from build123d import *

# Parameters (mm, degrees)
BOSS_EXTRUDE1_DEPTH                             = 3
BOSS_EXTRUDE2_START                             = 10
SKETCH2_R                                       = 2
BOSS_EXTRUDE2_DEPTH                             = 10
FILLET2_R                                       = 2
CSK_FOR_M3_FLAT_HEAD_MACHINE_SCREW1_D           = 3.2
CSK_FOR_M3_FLAT_HEAD_MACHINE_SCREW1_CSINK_D     = 6.3
CSK_FOR_M3_FLAT_HEAD_MACHINE_SCREW1_CSINK_ANGLE = 90
BOSS_EXTRUDE3_DEPTH                             = 2
BOSS_EXTRUDE3_DEPTH_BACK                        = 4
SKETCH5_W                                       = 113
SKETCH5_H                                       = 2
SKETCH5_W_2                                     = 2
SKETCH5_H_2                                     = 58
CHAMFER1_SIZE                                   = 2
CHAMFER2_SIZE                                   = 0.5
SKETCH6_R                                       = 1.75
CUT_EXTRUDE1_DEPTH                              = 86.283351383
SKETCH7_R                                       = 4
SKETCH7_R_2                                     = 2.75
BOSS_EXTRUDE4_DEPTH                             = 1.5
CUT_EXTRUDE2_START                              = -4
SKETCH8_R                                       = 2.75
CUT_EXTRUDE2_DEPTH                              = 4


with BuildPart() as part:
    # Sketch1 → Boss-Extrude1 (new body)
    with BuildSketch(Plane.XY):
        with BuildLine():
            Line((-66.5, 44), (66.5, 44))
            ThreePointArc((66.5, 44), (70.035533906, 42.535533906), (71.5, 39))
            Line((71.5, 39), (71.5, -39))
            ThreePointArc((71.5, -39), (70.035533906, -42.535533906), (66.5, -44))
            Line((66.5, -44), (-66.5, -44))
            ThreePointArc((-66.5, -44), (-70.035533906, -42.535533906), (-71.5, -39))
            Line((-71.5, -39), (-71.5, 39))
            ThreePointArc((-71.5, 39), (-70.035533906, 42.535533906), (-66.5, 44))
        make_face()
    extrude(amount=BOSS_EXTRUDE1_DEPTH)

    # Sketch2 → Boss-Extrude2 (add)
    with BuildSketch(Plane(origin=(0, 0, 0), x_dir=(-1, 0, 0), z_dir=(0, 0, -1)).offset(BOSS_EXTRUDE2_START)):
        with BuildLine():
            Line((-66.5, 44), (66.5, 44))
            ThreePointArc((66.5, 44), (70.035533906, 42.535533906), (71.5, 39))
            Line((71.5, 39), (71.5, -39))
            ThreePointArc((71.5, -39), (70.035533906, -42.535533906), (66.5, -44))
            Line((66.5, -44), (-66.5, -44))
            ThreePointArc((-66.5, -44), (-70.035533906, -42.535533906), (-71.5, -39))
            Line((-71.5, -39), (-71.5, 39))
            ThreePointArc((-71.5, 39), (-70.035533906, 42.535533906), (-66.5, 44))
        make_face()
        with Locations((-66.5, 39)):
            Circle(SKETCH2_R, mode=Mode.SUBTRACT)
        with Locations(Location((66.5, 39, 0), (0, 0, 180))):
            Circle(SKETCH2_R, mode=Mode.SUBTRACT)
        with Locations((66.5, -39)):
            Circle(SKETCH2_R, mode=Mode.SUBTRACT)
        with Locations(Location((-66.5, -39, 0), (0, 0, 180))):
            Circle(SKETCH2_R, mode=Mode.SUBTRACT)
        with BuildLine():
            Line((-61.917424305, 41), (61.917424305, 41))
            Line((61.917424305, 41), (61.917424305, 37))
            ThreePointArc((61.917424305, 37), (64.673843213, 34.345416088), (68.5, 34.417424305))
            Line((68.5, 34.417424305), (68.5, -34.417424305))
            ThreePointArc((68.5, -34.417424305), (64.673843213, -34.345416088), (61.917424305, -37))
            Line((61.917424305, -37), (61.917424305, -41))
            Line((61.917424305, -41), (-61.917424305, -41))
            ThreePointArc((-61.917424305, -41), (-62.964466094, -35.464466094), (-68.5, -34.417424305))
            Line((-68.5, -34.417424305), (-68.5, 34.417424305))
            ThreePointArc((-68.5, 34.417424305), (-62.964466094, 35.464466094), (-61.917424305, 41))
        make_face(mode=Mode.SUBTRACT)
    extrude(amount=-BOSS_EXTRUDE2_DEPTH)

    # Fillet2
    fillet2_edges = [part.edges().sort_by_distance(p)[0] for p in [
        (-70.035533906, -42.535533906, 3),
        (0, -44, 3),
        (70.035533906, -42.535533906, 3),
        (71.5, 0, 3),
        (70.035533906, 42.535533906, 3),
        (0, 44, 3),
        (0, 41, 0),
        (68.5, 0, 0),
        (0, -41, 0),
        (-68.5, 0, 0),
        (-70.035533906, 42.535533906, 3),
        (-71.5, 0, 3),
    ]]
    fillet(fillet2_edges, radius=FILLET2_R)

    # CSK for M3 Flat Head Machine Screw1 (through all)
    with Locations(Plane.XY.offset(3)):
        with Locations((-66.5, 39), (66.5, 39), (66.5, -39), (-66.5, -39)):
            CounterSinkHole(CSK_FOR_M3_FLAT_HEAD_MACHINE_SCREW1_D / 2, CSK_FOR_M3_FLAT_HEAD_MACHINE_SCREW1_CSINK_D / 2, counter_sink_angle=CSK_FOR_M3_FLAT_HEAD_MACHINE_SCREW1_CSINK_ANGLE)

    # Sketch5 → Boss-Extrude3 (add, two sides: drawn at the far end of the back side and taken through both)
    with BuildSketch(Plane(origin=(0, 0, -10), x_dir=(-1, 0, 0), z_dir=(0, 0, -1)).offset(-BOSS_EXTRUDE3_DEPTH_BACK)):
        with Locations((0, 40)):
            Rectangle(SKETCH5_W, SKETCH5_H)
        with Locations((-67.5, 0)):
            Rectangle(SKETCH5_W_2, SKETCH5_H_2)
        with Locations((0, -40)):
            Rectangle(SKETCH5_W, SKETCH5_H)
        with Locations((67.5, 0)):
            Rectangle(SKETCH5_W_2, SKETCH5_H_2)
    extrude(amount=BOSS_EXTRUDE3_DEPTH + BOSS_EXTRUDE3_DEPTH_BACK)

    # Chamfer1
    chamfer1_edges = [part.edges().sort_by_distance(p)[0] for p in [
        (0, -39, -6),
        (-66.5, 0, -6),
        (66.5, 0, -6),
        (0, 39, -6),
    ]]
    chamfer(chamfer1_edges, length=CHAMFER1_SIZE - 0.0001)  # a hair under: the kernel refuses the full size

    # Chamfer2
    chamfer2_edges = [part.edges().sort_by_distance(p)[0] for p in [
        (0, 41, -12),
        (68.5, 0, -12),
        (0, -41, -12),
        (-68.5, 0, -12),
    ]]
    chamfer(chamfer2_edges, length=CHAMFER2_SIZE)

    # Sketch6 → Cut-Extrude1 (cut, through all)
    with BuildSketch(Plane.XY.offset(3)):
        with Locations((-50, 23.5)):
            Circle(SKETCH6_R)
        with Locations((-50, -3.5)):
            Circle(SKETCH6_R)
        with Locations((50, -3.5)):
            Circle(SKETCH6_R)
        with Locations((50, 23.5)):
            Circle(SKETCH6_R)
    extrude(amount=-CUT_EXTRUDE1_DEPTH, mode=Mode.SUBTRACT)

    # Sketch7 → Boss-Extrude4 (add)
    # profile 1 of 4: a face of its own
    with BuildSketch(Plane(origin=(0, 0, 0), x_dir=(-1, 0, 0), z_dir=(0, 0, -1))):
        with Locations(Location((-50, 23.5, 0), (0, 0, 180))):
            Circle(SKETCH7_R)
        with Locations((-50, 23.5)):
            Circle(SKETCH7_R_2, mode=Mode.SUBTRACT)
    # profile 2 of 4: a face of its own
    with BuildSketch(Plane(origin=(0, 0, 0), x_dir=(-1, 0, 0), z_dir=(0, 0, -1))):
        with Locations(Location((-50, -3.5, 0), (0, 0, 180))):
            Circle(SKETCH7_R)
        with Locations((-50, -3.5)):
            Circle(SKETCH7_R_2, mode=Mode.SUBTRACT)
    # profile 3 of 4: a face of its own
    with BuildSketch(Plane(origin=(0, 0, 0), x_dir=(-1, 0, 0), z_dir=(0, 0, -1))):
        with Locations(Location((50, -3.5, 0), (0, 0, 180))):
            Circle(SKETCH7_R)
        with Locations((50, -3.5)):
            Circle(SKETCH7_R_2, mode=Mode.SUBTRACT)
    # profile 4 of 4: a face of its own
    with BuildSketch(Plane(origin=(0, 0, 0), x_dir=(-1, 0, 0), z_dir=(0, 0, -1))):
        with Locations(Location((50, 23.5, 0), (0, 0, 180))):
            Circle(SKETCH7_R)
        with Locations((50, 23.5)):
            Circle(SKETCH7_R_2, mode=Mode.SUBTRACT)
    extrude(amount=BOSS_EXTRUDE4_DEPTH)

    # Sketch8 → Cut-Extrude2 (cut)
    with BuildSketch(Plane(origin=(0, 0, -1.5), x_dir=(-1, 0, 0), z_dir=(0, 0, -1)).offset(CUT_EXTRUDE2_START)):
        with Locations((-50, 23.5)):
            Circle(SKETCH8_R)
        with Locations((-50, -3.5)):
            Circle(SKETCH8_R)
        with Locations((50, -3.5)):
            Circle(SKETCH8_R)
        with Locations((50, 23.5)):
            Circle(SKETCH8_R)
    extrude(amount=CUT_EXTRUDE2_DEPTH, mode=Mode.SUBTRACT)


solid = part.part
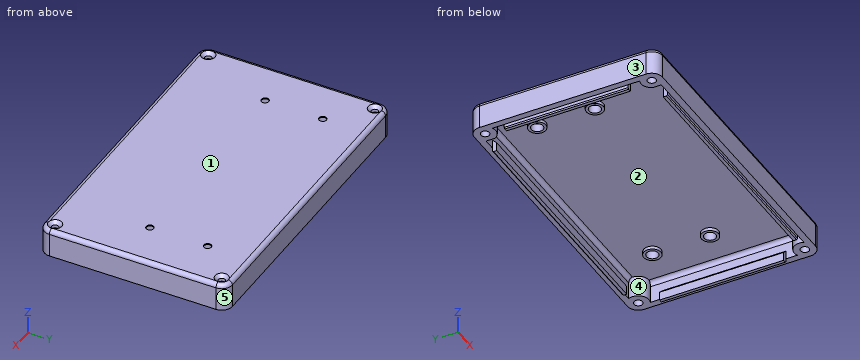
Verification items for the finished model (mm, model axes). Face numbers are marked on the shaded views. A direction names the side the tool comes from. Coordinates: 2 decimals unless noted, no trailing zeros. Loops run counter-clockwise (first coordinate to the right, second up) from the corner with the lowest first, then second, coordinate; pieces in that order, holes last. Notation, with made-up numbers: (-31, 59) -> (9, 59) arc R29 ccw to (9, 81) -> close; hole circle Ø6 at (66.5, 62). An arc over 180 degrees is marked (long way). Answer as a JSON object with one key per item and string values. Group by question number.
Item 1: Tool access check on the marked faces 1 and 2. Record the directions out of +Z, -Z, +X, -X, +Y, -Y that give a thin tool (end or side, any length) a straight path to the whole face; none if there is none.
Item 2: Scan lines: probe 1 along Y at (x, z) = (66.5, -2.25); probe 2 along X at (y, z) = (-17.5, -2.75); probe 3 along X at (y, z) = (6, -6.5). Record each from-to range of solid material in increasing order.
Item 3: Depth check by flat-ended pin: pin 1 (3 mm diameter, centred on x = -39, y = -33.5, fed in from -Z); pin 2 (4.5 mm diameter, centred on x = 66, y = 40, fed in from -Z); pin 3 (1.6 mm diameter, centred on x = -51.5, y = 22.5, fed in from -Z). Enter the tip coordinate at first touch or a pass-through.
Item 4: Sectioned sample at B-B on x = 50. State how many separate pieces and enclosed holes the cut face has, plus the area to 3 significant figures.
Item 5: Mould release check, pull along Y, two halves, no side actions. Record for the marked faces 3, 4 and 5: +Y half, -Y half, draft (parallel to the pull), parting line (faces both ways), or undercut.
Item 6: Sectioned sample at D-D on y = -31. Record the boundary of the cut face in (x, z).
Evaluation:
{
 "1": {"face 1": "+Z, +X, -X, +Y, -Y", "face 2": "-Z"},
 "2": {"probe 1": "y = -44 to -41, -37 to -34, 34 to 37, 41 to 44", "probe 2": "x = -71.5 to -68.5, 68.5 to 71.5", "probe 3": "x = -71.5 to -68, 68 to 71.5"},
 "3": {"pin 1": "stops at z = 0", "pin 2": "stops at z = -10", "pin 3": "stops at z = 2.5"},
 "4": {"separate pieces": "3", "enclosed holes": "0", "area": "320 mm²"},
 "5": {"face 3": "draft", "face 4": "undercut", "face 5": "+Y half"},
 "6": {"outline": "(-71.5, -10) -> (-68.5, -10) -> (-68.5, -2) arc R2 cw to (-66.5, 0) -> (66.5, 0) arc R2 cw to (68.5, -2) -> (68.5, -10) -> (71.5, -10) -> (71.5, 1) arc R2 ccw to (69.5, 3) -> (-69.5, 3) arc R2 ccw to (-71.5, 1) -> close"}
}
